from build123d import *

# Parameters (mm, degrees)
EXTRUSION1_DEPTH = 32
ESQUISSE2_R      = 1.5
EXTRUSION2_DEPTH = 25
ESQUISSE3_R      = 1.5
EXTRUSION3_DEPTH = 25


with BuildPart() as part:
    # Esquisse1 → Extrusion1 (new body)
    with BuildSketch(Plane.XY):
        Polygon((-12.537924369, 4.331190223), (-12.537924369, -10.668809777), (2.462075631, -10.668809777), (2.462075631, -9.168809777), (-11.037924369, -9.168809777), (-11.037924369, 4.331190223), align=None)
    extrude(amount=EXTRUSION1_DEPTH)

    # Esquisse2 → Extrusion2 (cut)
    with BuildSketch(Plane.ZY.offset(12.537924369)):
        with Locations(Location((23, -3.168809777, 0), (0, 0, 270))):
            Circle(ESQUISSE2_R)
        with Locations(Location((5, -3.168809777, 0), (0, 0, 270))):
            Circle(ESQUISSE2_R)
    extrude(amount=-EXTRUSION2_DEPTH, mode=Mode.SUBTRACT)

    # Esquisse3 → Extrusion3 (cut)
    with BuildSketch(Plane.XZ.offset(10.668809777)):
        with Locations(Location((-5.037924369, 5, 0), (0, 0, 270))):
            Circle(ESQUISSE3_R)
        with Locations(Location((-5.037924369, 27, 0), (0, 0, 270))):
            Circle(ESQUISSE3_R)
        with Locations(Location((-5.037924369, 16, 0), (0, 0, 270))):
            Circle(ESQUISSE3_R)
    extrude(amount=-EXTRUSION3_DEPTH, mode=Mode.SUBTRACT)


solid = part.part
Geometry check sheet. Reference: the model listing, model coordinates, mm. Give positions to 0.01 mm unless a question says otherwise; leave off trailing zeros. Order: outer loops, then holes, each group sorted by start corner. A loop starts at its lowest first (then second) coordinate and runs counter-clockwise, first axis right, second up.
1. Draft check along X on faces 1 (the face through (-11.038, -3, 16)), 2 (the face through (-5, -9.9, 17.5)), 3 (the face through (-3, -9.169, 16)). Enter one of: pulls with the +X half, pulls with the -X half, needs draft (parallel to the pull), parting line crosses it, or undercut.
Completed:
face 1: pulls with the +X half
face 2: undercut
face 3: needs draft
2. Sectioned sample at D-D (x = -4.5). Record the boundary of the cut face in (y, z).
Completed:
outline: (-10.67, 0) - (-9.17, 0) - (-9.17, 3.6) - (-10.67, 3.6) - close; (-10.67, 6.4) - (-9.17, 6.4) - (-9.17, 14.6) - (-10.67, 14.6) - close; (-10.67, 17.4) - (-9.17, 17.4) - (-9.17, 25.6) - (-10.67, 25.6) - close; (-10.67, 28.4) - (-9.17, 28.4) - (-9.17, 32) - (-10.67, 32) - close
3. Depth check by flat-ended pin: pin 1 (6 mm diameter, centred on y = -1, z = 23, fed in from +X); pin 2 (3.5 mm diameter, centred on x = -5.04, z = 27, fed in from +Y). Enter the tip coordinate at first touch or a pass-through.
Completed:
pin 1: stops at x = -11.04
pin 2: stops at y = -9.17
4. Sectioned sample at C-C (z = 5). Record the boundary of the cut face in (x, y), then the cut area to 4 significant figures.
Completed:
outline: (-12.54, -10.67) - (-6.54, -10.67) - (-6.54, -9.17) - (-11.04, -9.17) - (-11.04, -4.67) - (-12.54, -4.67) - close; (-12.54, -1.67) - (-11.04, -1.67) - (-11.04, 4.33) - (-12.54, 4.33) - close; (-3.54, -10.67) - (2.46, -10.67) - (2.46, -9.17) - (-3.54, -9.17) - close
area: 33.75 mm2
5. Sectioned sample at B-B (y = -2). Record the boundary of the cut face in (x, z), then the cut area to 3 significant figures.
Completed:
outline: (-12.54, 0) - (-11.04, 0) - (-11.04, 4.06) - (-12.54, 4.06) - close; (-12.54, 5.94) - (-11.04, 5.94) - (-11.04, 22.06) - (-12.54, 22.06) - close; (-12.54, 23.94) - (-11.04, 23.94) - (-11.04, 32) - (-12.54, 32) - close
area: 42.4 mm2
6. Scan lines: line 1 (X direction, y = -10.05, z = 27); line 2 (Y direction, x = -8, z = 18.5); line 3 (X direction, y = -6.25, z = 3). Record each from-to range of solid material in increasing order.
Completed:
line 1: x = -12.54 to -6.54, -3.54 to 2.46
line 2: y = -10.67 to -9.17
line 3: x = -12.54 to -11.04
7. Sectioned sample at A-A (z = 23). Record the boundary of the cut face in (x, y), then the cut area to 4 significant figures.
Completed:
outline: (-12.54, -10.67) - (2.46, -10.67) - (2.46, -9.17) - (-11.04, -9.17) - (-11.04, -4.67) - (-12.54, -4.67) - close; (-12.54, -1.67) - (-11.04, -1.67) - (-11.04, 4.33) - (-12.54, 4.33) - close
area: 38.25 mm2
